Build history of the part. All positions in model axes, mm. A direction names the side the tool comes from. Round coordinates to 2 decimals unless told otherwise and drop trailing zeros. Write each loop counter-clockwise with the first axis right and the second up, starting at its lowest first coordinate (ties: lowest second). Pieces come first, ordered by that corner, then holes. Notation, with made-up numbers: M -35.75,43.25 L 11.25,43.25 A13 ccw 11.25,54.25 Z; hole C -16,65.25 d2. An arc over 180 degrees is marked long. Use a Markdown table: item, result.
from build123d import *

# Parameters (mm, degrees)
F1_DEPTH = 127


with BuildPart() as f1:
    # F0 (on Front) → F1 (new body)
    with BuildSketch(Plane.XZ):
        with BuildLine():
            Line((0, 38.1), (0, -38.1))
            Line((0, -38.1), (33.02, -38.1))
            ThreePointArc((33.02, -38.1), (35.12925, -35.596791), (33.02, -33.093582))
            Line((33.02, -33.093582), (8.555139, -29.970825))
            ThreePointArc((8.555139, -29.970825), (5.528239, -28.364406), (4.318, -25.158469))
            Line((4.318, -25.158469), (4.318, 0))
            Line((4.318, 0), (4.318, 25.158469))
            ThreePointArc((4.318, 25.158469), (5.528239, 28.364406), (8.555139, 29.970825))
            Line((8.555139, 29.970825), (33.02, 33.093582))
            ThreePointArc((33.02, 33.093582), (35.12925, 35.596791), (33.02, 38.1))
            Line((33.02, 38.1), (0, 38.1))
        make_face()
    extrude(amount=F1_DEPTH)


solid = f1.part
Q1. Cut at C-C on z = 19. Give the cut face in (x, y), and give its area (3 significant figures).
Response values:
| item | result |
|---|---|
| outline | M 0,-127 L 4.32,-127 L 4.32,0 L 0,0 Z |
| area | 548 mm2 |
Q2. Cut at A-A on y = -67. Give the cut face in (x, z), and give its area (3 significant figures).
Response values:
| item | result |
|---|---|
| outline | M 0,-38.1 L 33.02,-38.1 A2.54 ccw 33.02,-33.09 L 8.56,-29.97 A4.85 cw 4.32,-25.16 L 4.32,25.16 A4.85 cw 8.56,29.97 L 33.02,33.09 A2.54 ccw 33.02,38.1 L 0,38.1 Z |
| area | 745 mm2 |
Q3. Cut at B-B on x = 24.5. Give the cut face in (y, z).
Response values:
| item | result |
|---|---|
| outline | M -127,-38.1 L 0,-38.1 L 0,-32.01 L -127,-32.01 Z; M -127,32.01 L 0,32.01 L 0,38.1 L -127,38.1 Z |
Q4. Which spindle directions (+Z, -Z, +X, -X, +Y, -Y) get a long thin tool onto all of the face, cutting with end or side? Do faces 4 (the flat face through (4.318, -63, 0)), 5 (the flat face through (3, 0, 3)). Say none if no direction does.
Response values:
| item | result |
|---|---|
| face 4 | +X, +Y, -Y |
| face 5 | +Z, -Z, +X, -X, +Y |
Q5. Cut at D-D on z = -27. Give the cut face in (x, y), and give its area (4 significant figures).
Response values:
| item | result |
|---|---|
| outline | M 0,-127 L 4.68,-127 L 4.68,0 L 0,0 Z |
| area | 594.5 mm2 |
Q6. Drop flat-ended pins along their axis: P1, Ø10, axis at x = 10.5, z = -0.5, coming from the -Y side; P2, Ø12, axis at y = -90.5, z = 14.5, coming from the +X side. Give the stop position or say it passes through.
Response values:
| item | result |
|---|---|
| P1 | passes through |
| P2 | stops at x = 4.32 |
Q7. Drill centre lines: L1, parallel to X at y = -16, z = -13; L2, parallel to Z at x = 17, y = -8; L3, parallel to Z at x = 24, y = -16. Where is each one in solid material? Low to high.
Response values:
| item | result |
|---|---|
| L1 | x = 0 to 4.32 |
| L2 | z = -38.1 to -31.05, 31.05 to 38.1 |
| L3 | z = -38.1 to -31.94, 31.94 to 38.1 |
Q8. Two-plate mould, pull along Z, no slides. Class faces 1 (the cylindrical face through (5.5, -62.61, 28.33)), 2 (the flat face through (0, -63, 1)), 3 (the flat face through (17, -63, 38.1)): +Z half, -Z half, draft (parallel to the pull), parting line (faces both ways), or undercut.
Response values:
| item | result |
|---|---|
| face 1 | undercut |
| face 2 | draft |
| face 3 | +Z half |
